```python
from build123d import *

# Parameters (mm, degrees)
SKETCH1_W           = 64.012274628
SKETCH1_H           = 75.085000506
BOSS_EXTRUDE1_DEPTH = 5
SKETCH7_R           = 1.4732
CUT_EXTRUDE1_DEPTH  = 10
SKETCH8_R           = 1.5
BOSS_EXTRUDE2_DEPTH = 2


with BuildPart() as part:
    # Sketch1 → Boss-Extrude1 (new body)
    # profile 1 of 2: a face of its own
    with BuildSketch(Plane.XY):
        with Locations((61.398411242, 7.077500224)):
            Rectangle(SKETCH1_W, SKETCH1_H)
        with BuildLine():
            ThreePointArc((83.484398078, 2.429730903), (59.871437613, -17.479677368), (44.238109553, 9.157805497))
            ThreePointArc((44.238109553, 9.157805497), (59.81501285, 35.930775127), (83.520814038, 15.994205484))
            ThreePointArc((83.520814038, 15.994205484), (83.22114917, 12.52456978), (82.331029644, 9.157693158))
            ThreePointArc((82.331029644, 9.157693158), (83.193968093, 5.842784333), (83.484398078, 2.429730903))
        make_face(mode=Mode.SUBTRACT)
    # profile 2 of 2: a face of its own
    with BuildSketch(Plane.XY):
        with Locations((-2.613863386, 7.077500224)):
            Rectangle(SKETCH1_W, SKETCH1_H)
        with BuildLine():
            ThreePointArc((15.69984642, 2.429730903), (-7.913055331, -17.479687433), (-23.546481788, 9.157693158))
            ThreePointArc((-23.546481788, 9.157693158), (-7.969677608, 35.930764895), (15.736182375, 15.994205484))
            ThreePointArc((15.736182375, 15.994205484), (15.436527739, 12.524628574), (14.546438303, 9.157805497))
            ThreePointArc((14.546438303, 9.157805497), (15.409406369, 5.842843047), (15.69984642, 2.429730903))
        make_face(mode=Mode.SUBTRACT)
    extrude(amount=BOSS_EXTRUDE1_DEPTH)

    # Sketch7 → Cut-Extrude1 (cut)
    with BuildSketch(Plane.XY.offset(5)):
        with Locations((-23.500584488, 33.499560055)):
            Circle(SKETCH7_R)
        with Locations((14.49941543, 33.50027263)):
            Circle(SKETCH7_R)
        with Locations((-23.49959354, -19.345440441)):
            Circle(SKETCH7_R)
        with Locations((14.500406379, -19.344727866)):
            Circle(SKETCH7_R)
        with Locations((44.284829686, -19.345328379)):
            Circle(SKETCH7_R)
        with Locations((44.284150424, 33.499672122)):
            Circle(SKETCH7_R)
        with Locations((82.284150347, 33.500160568)):
            Circle(SKETCH7_R)
        with Locations((82.284829608, -19.344839933)):
            Circle(SKETCH7_R)
    extrude(amount=-CUT_EXTRUDE1_DEPTH, mode=Mode.SUBTRACT)

    # Sketch8 → Boss-Extrude2 (add)
    # profile 1 of 2: a face of its own
    with BuildSketch(Plane(origin=(0, 0, 0), x_dir=(-1, 0, 0), z_dir=(0, 0, -1))):
        with BuildLine():
            ThreePointArc((-44.238109553, 9.157805497), (-63.284649438, 36.230429762), (-82.331029644, 9.157693158))
            ThreePointArc((-82.331029644, 9.157693158), (-63.284490186, -17.770117418), (-44.238109553, 9.157805497))
        make_face()
        with Locations((-63.284549757, 2.429730903)):
            Circle(SKETCH8_R, mode=Mode.SUBTRACT)
        with Locations((-63.28458976, 15.994205484)):
            Circle(SKETCH8_R, mode=Mode.SUBTRACT)
    # profile 2 of 2: a face of its own
    with BuildSketch(Plane(origin=(0, 0, 0), x_dir=(-1, 0, 0), z_dir=(0, 0, -1))):
        with BuildLine():
            ThreePointArc((23.546481788, 9.157693158), (4.500101582, 36.230429762), (-14.546438303, 9.157805497))
            ThreePointArc((-14.546438303, 9.157805497), (4.49994233, -17.770117418), (23.546481788, 9.157693158))
        make_face()
        with Locations((4.500041904, 15.994205484)):
            Circle(SKETCH8_R, mode=Mode.SUBTRACT)
        with Locations((4.500001901, 2.429730903)):
            Circle(SKETCH8_R, mode=Mode.SUBTRACT)
    extrude(amount=-BOSS_EXTRUDE2_DEPTH)


solid = part.part
```
Verification items for the finished model (mm, model axes). A direction names the side the tool comes from. Round coordinates to 2 decimals unless told otherwise and drop trailing zeros. Write each loop counter-clockwise with the first axis right and the second up, starting at its lowest first coordinate (ties: lowest second). Pieces come first, ordered by that corner, then holes. Notation, with made-up numbers: (-1.5, 16) - (3.5, 16) arc R16 cw to (3.5, 43) - close; hole circle Ø11 at (-14.5, 77.25). An arc over 180 degrees is marked (long way). Answer as a JSON object with one key per item and string values. Group by question number.
Q1. Section check D-D, the plane x = -13. Enter the section's corners in (y, z) (3 decimals).
Q2. Section check A-A, the plane z = 3.15. Give the number of separate pieces and of enclosed holes in the cut face, plus the area to 3 significant figures.
Q3. Section check B-B, the plane y = 27. Enter the section's corners in (x, z), plus the area to 3 significant figures.
Q4. Thickness scan on line 1 (X direction, y = -19.5, z = 2.35); line 2 (X direction, y = 33.5, z = 1.35); line 3 (X direction, y = 15, z = 4.5). Record the ranges inside material, lowest first.
Q5. Go/stop test with flat-tipped pins: pin 1 Ø24.5 at (x, y) = (63.28, 15.99) entering from +Z; pin 2 Ø2.5 at (x, y) = (14.5, -19.34) entering from -Z. Record where each tip stops, or that it passes through.
Q6. Tool access check on faces 1 (the flat face through (64, 10, 2)), 2 (the cylindrical face through (61.854, 16.445, 0.986)). Record the directions out of +Z, -Z, +X, -X, +Y, -Y that give a thin tool (end or side, any length) a straight path to the whole face; none if there is none.
Q7. Mould release check, pull along Y, two halves, no side actions. Record for faces 3 (the flat face through (30, 8, 0)), 4 (the cylindrical face through (-3.31, 1.517, 0.986)), 5 (the flat face through (28, -30.465, 2)): released by +Y, released by -Y, zero draft, split by the parting line, or undercut.
Q8. Section check C-C, the plane x = 76. Enter the section's corners in (y, z) (3 decimals).
Found:
{
 "1": {"outline": "(-30.465, 0) - (44.62, 0) - (44.62, 5) - (34.359, 5) - (34.359, 2) - (-15.895, 2) - (-15.895, 5) - (-30.465, 5) - close"},
 "2": {"separate pieces": "1", "enclosed holes": "10", "area": "5,910 mm^2"},
 "3": {"outline": "(-34.62, 0) - (93.4, 0) - (93.4, 5) - (80.27, 5) - (80.27, 2) - (46.3, 2) - (46.3, 5) - (12.48, 5) - (12.48, 2) - (-21.48, 2) - (-21.48, 5) - (-34.62, 5) - close", "area": "436 mm^2"},
 "4": {"line 1": "x = -34.62 to -24.96, -22.03 to 13.04, 15.97 to 42.82, 45.75 to 80.82, 83.75 to 93.4", "line 2": "x = -34.62 to -24.97, -22.03 to 13.03, 15.97 to 42.81, 45.76 to 80.81, 83.76 to 93.4", "line 3": "x = -34.62 to -24.71, 15.71 to 43.07, 83.5 to 93.4"},
 "5": {"pin 1": "stops at z = 2", "pin 2": "passes through"},
 "6": {"face 1": "+Z", "face 2": "+Z, -Z"},
 "7": {"face 3": "zero draft", "face 4": "undercut", "face 5": "released by -Y"},
 "8": {"outline": "(-30.465, 0) - (44.62, 0) - (44.62, 5) - (31.737, 5) - (31.737, 2) - (-13.266, 2) - (-13.266, 5) - (-30.465, 5) - close"}
}
